Check sheet for the modelled part. Datum: model origin and axes. Units: mm. A direction names the side the tool comes from. Give positions to 0.01 mm unless a question says otherwise; leave off trailing zeros. Order: outer loops, then holes, each group sorted by start corner. A loop starts at its lowest first (then second) coordinate and runs counter-clockwise, first axis right, second up.
```python
from build123d import *

# Parameters (mm, degrees)
BOSS_EXTRUDE1_DEPTH = 3
CUT_EXTRUDE1_REACH  = 77.661
SKETCH1_3_R         = 1.25
BOSS_EXTRUDE2_START = 8.86
BOSS_EXTRUDE2_DEPTH = 8.86
BOSS_EXTRUDE3_START = 1.5
SKETCH1_5_R         = 3.21
SKETCH1_5_R_2       = 1.25
BOSS_EXTRUDE3_DEPTH = 1.5
SKETCH2_W           = 12.28
SKETCH2_H           = 8.73
CUT_EXTRUDE2_DEPTH  = 3
SKETCH3_R           = 1.6
BOSS_EXTRUDE4_DEPTH = 3
FILLET1_R           = 1
FILLET2_R           = 1


with BuildPart() as part:
    # Sketch1 → Boss-Extrude1 (new body)
    with BuildSketch(Plane(origin=(0, 0, 0), x_dir=(1, 0, 0), z_dir=(0, 1, 0))):
        with BuildLine():
            Line((3.81, 3), (49.09, 3))
            ThreePointArc((49.09, 3), (53.90539718, 1.00539718), (55.9, -3.81))
            Line((55.9, -3.81), (55.9, -44.09))
            ThreePointArc((55.9, -44.09), (53.90539718, -48.90539718), (49.09, -50.9))
            Line((49.09, -50.9), (3.81, -50.9))
            ThreePointArc((3.81, -50.9), (-1.00539718, -48.90539718), (-3, -44.09))
            Line((-3, -44.09), (-3, -3.81))
            ThreePointArc((-3, -3.81), (-1.00539718, 1.00539718), (3.81, 3))
        make_face()
    extrude(amount=-BOSS_EXTRUDE1_DEPTH)

    # Sketch1_3 → Cut-Extrude1 (cut, up to next)
    with BuildSketch(Plane(origin=(0, 0, 0), x_dir=(1, 0, 0), z_dir=(0, 1, 0)), mode=Mode.PRIVATE) as cut_extrude1_sk1:
        with Locations(Location((3.81, -3.81, 0), (0, 0, 270))):
            Circle(SKETCH1_3_R)
    cut_extrude1_tool1 = extrude(cut_extrude1_sk1.sketch, amount=-CUT_EXTRUDE1_REACH, mode=Mode.PRIVATE) & part.part
    # Sketch1_3 → Cut-Extrude1 (cut, up to next)
    with BuildSketch(Plane(origin=(0, 0, 0), x_dir=(1, 0, 0), z_dir=(0, 1, 0)), mode=Mode.PRIVATE) as cut_extrude1_sk2:
        with Locations(Location((3.81, -44.09, 0), (0, 0, 270))):
            Circle(SKETCH1_3_R)
    cut_extrude1_tool2 = extrude(cut_extrude1_sk2.sketch, amount=-CUT_EXTRUDE1_REACH, mode=Mode.PRIVATE) & part.part
    # Sketch1_3 → Cut-Extrude1 (cut, up to next)
    with BuildSketch(Plane(origin=(0, 0, 0), x_dir=(1, 0, 0), z_dir=(0, 1, 0)), mode=Mode.PRIVATE) as cut_extrude1_sk3:
        with Locations(Location((49.09, -44.09, 0), (0, 0, 270))):
            Circle(SKETCH1_3_R)
    cut_extrude1_tool3 = extrude(cut_extrude1_sk3.sketch, amount=-CUT_EXTRUDE1_REACH, mode=Mode.PRIVATE) & part.part
    # Sketch1_3 → Cut-Extrude1 (cut, up to next)
    with BuildSketch(Plane(origin=(0, 0, 0), x_dir=(1, 0, 0), z_dir=(0, 1, 0)), mode=Mode.PRIVATE) as cut_extrude1_sk4:
        with Locations(Location((49.09, -3.81, 0), (0, 0, 270))):
            Circle(SKETCH1_3_R)
    cut_extrude1_tool4 = extrude(cut_extrude1_sk4.sketch, amount=-CUT_EXTRUDE1_REACH, mode=Mode.PRIVATE) & part.part
    add(cut_extrude1_tool1.solids().sort_by_distance((3.81, 0, 3.81))[0], mode=Mode.SUBTRACT)
    add(cut_extrude1_tool2.solids().sort_by_distance((3.81, 0, 44.09))[0], mode=Mode.SUBTRACT)
    add(cut_extrude1_tool3.solids().sort_by_distance((49.09, 0, 44.09))[0], mode=Mode.SUBTRACT)
    add(cut_extrude1_tool4.solids().sort_by_distance((49.09, 0, 3.81))[0], mode=Mode.SUBTRACT)

    # Sketch1_4 → Boss-Extrude2 (add)
    with BuildSketch(Plane(origin=(0, 0, 0), x_dir=(1, 0, 0), z_dir=(0, 1, 0)).offset(BOSS_EXTRUDE2_START)):
        with BuildLine():
            ThreePointArc((-3, -3.81), (-1.00539718, 1.00539718), (3.81, 3))
            Line((3.81, 3), (49.09, 3))
            ThreePointArc((49.09, 3), (53.90539718, 1.00539718), (55.9, -3.81))
            Line((55.9, -3.81), (55.9, -44.09))
            ThreePointArc((55.9, -44.09), (53.90539718, -48.90539718), (49.09, -50.9))
            Line((49.09, -50.9), (3.81, -50.9))
            ThreePointArc((3.81, -50.9), (-1.00539718, -48.90539718), (-3, -44.09))
            Line((-3, -44.09), (-3, -3.81))
        make_face()
        with BuildLine():
            Line((52.9, -3.81), (52.9, -44.09))
            ThreePointArc((52.9, -44.09), (51.784076836, -46.784076836), (49.09, -47.9))
            Line((49.09, -47.9), (3.81, -47.9))
            ThreePointArc((3.81, -47.9), (1.115923164, -46.784076836), (0, -44.09))
            Line((0, -44.09), (0, -3.81))
            ThreePointArc((0, -3.81), (1.115923164, -1.115923164), (3.81, 0))
            Line((3.81, 0), (49.09, 0))
            ThreePointArc((49.09, 0), (51.784076836, -1.115923164), (52.9, -3.81))
        make_face(mode=Mode.SUBTRACT)
    extrude(amount=-BOSS_EXTRUDE2_DEPTH)

    # Sketch1_5 → Boss-Extrude3 (add)
    # profile 1 of 4: a face of its own
    with BuildSketch(Plane(origin=(0, 0, 0), x_dir=(1, 0, 0), z_dir=(0, 1, 0)).offset(BOSS_EXTRUDE3_START)):
        with Locations(Location((49.09, -3.81, 0), (0, 0, 90))):
            Circle(SKETCH1_5_R)
        with Locations(Location((49.09, -3.81, 0), (0, 0, 270))):
            Circle(SKETCH1_5_R_2, mode=Mode.SUBTRACT)
    # profile 2 of 4: a face of its own
    with BuildSketch(Plane(origin=(0, 0, 0), x_dir=(1, 0, 0), z_dir=(0, 1, 0)).offset(BOSS_EXTRUDE3_START)):
        with Locations(Location((49.09, -44.09, 0), (0, 0, 90))):
            Circle(SKETCH1_5_R)
        with Locations(Location((49.09, -44.09, 0), (0, 0, 270))):
            Circle(SKETCH1_5_R_2, mode=Mode.SUBTRACT)
    # profile 3 of 4: a face of its own
    with BuildSketch(Plane(origin=(0, 0, 0), x_dir=(1, 0, 0), z_dir=(0, 1, 0)).offset(BOSS_EXTRUDE3_START)):
        with Locations(Location((3.81, -44.09, 0), (0, 0, 90))):
            Circle(SKETCH1_5_R)
        with Locations(Location((3.81, -44.09, 0), (0, 0, 270))):
            Circle(SKETCH1_5_R_2, mode=Mode.SUBTRACT)
    # profile 4 of 4: a face of its own
    with BuildSketch(Plane(origin=(0, 0, 0), x_dir=(1, 0, 0), z_dir=(0, 1, 0)).offset(BOSS_EXTRUDE3_START)):
        with Locations(Location((3.81, -3.81, 0), (0, 0, 90))):
            Circle(SKETCH1_5_R)
        with Locations(Location((3.81, -3.81, 0), (0, 0, 270))):
            Circle(SKETCH1_5_R_2, mode=Mode.SUBTRACT)
    extrude(amount=-BOSS_EXTRUDE3_DEPTH)

    # Sketch2 → Cut-Extrude2 (cut)
    with BuildSketch(Plane.XY.offset(50.9)):
        with Locations((18.5, 4.5)):
            Rectangle(SKETCH2_W, SKETCH2_H)
    extrude(amount=-CUT_EXTRUDE2_DEPTH, mode=Mode.SUBTRACT)

    # Sketch3 → Boss-Extrude4 (add)
    # profile 1 of 2: a face of its own
    with BuildSketch(Plane.XZ.offset(3)):
        with BuildLine():
            Line((55.9, 18.95), (62, 18.95))
            ThreePointArc((62, 18.95), (64.757716447, 20.092283553), (65.9, 22.85))
            Line((65.9, 22.85), (65.9, 25.05))
            ThreePointArc((65.9, 25.05), (64.757716447, 27.807716447), (62, 28.95))
            Line((62, 28.95), (55.9, 28.95))
            Line((55.9, 28.95), (55.9, 18.95))
        make_face()
        with Locations(Location((60.9, 23.95, 0), (0, 0, 270))):
            Circle(SKETCH3_R, mode=Mode.SUBTRACT)
    # profile 2 of 2: a face of its own
    with BuildSketch(Plane.XZ.offset(3)):
        with BuildLine():
            Line((-3, 18.95), (-9.1, 18.95))
            ThreePointArc((-9.1, 18.95), (-11.857716447, 20.092283553), (-13, 22.85))
            Line((-13, 22.85), (-13, 25.05))
            ThreePointArc((-13, 25.05), (-11.857716447, 27.807716447), (-9.1, 28.95))
            Line((-9.1, 28.95), (-3, 28.95))
            Line((-3, 28.95), (-3, 18.95))
        make_face()
        with Locations(Location((-8, 23.95, 0), (0, 0, 270))):
            Circle(SKETCH3_R, mode=Mode.SUBTRACT)
    extrude(amount=-BOSS_EXTRUDE4_DEPTH)

    # Fillet1
    fillet1_edges = [part.edges().sort_by_distance(p)[0] for p in [
        (58.95, 0, 28.95),
        (64.757716447, 0, 27.807716447),
        (65.9, 0, 23.95),
        (64.757716447, 0, 20.092283553),
        (58.95, 0, 18.95),
    ]]
    fillet(fillet1_edges, radius=FILLET1_R)

    # Fillet2
    fillet2_edges = [part.edges().sort_by_distance(p)[0] for p in [
        (-6.05, 0, 18.95),
        (-11.857716447, 0, 20.092283553),
        (-13, 0, 23.95),
        (-11.857716447, 0, 27.807716447),
        (-6.05, 0, 28.95),
    ]]
    fillet(fillet2_edges, radius=FILLET2_R)


solid = part.part
```
(1) Release check for a two-part mould opening along X. For faces 1 (the face through (64.727, -2.014, 20.062)), 2 (the face through (-9, -1.5, 25.2)), 3 (the face through (-13, -2, 24)), 4 (the face through (59, 0, 23)) record: released by +X, released by -X, zero draft, split by the parting line, or undercut.
Response values:
face 1: released by +X
face 2: undercut
face 3: released by -X
face 4: zero draft
(2) Material ranges on L1, parallel to X at y = -0.5, z = 3.81; L2, parallel to X at y = -1.55, z = 23.95; L3, parallel to Z at x = 4, y = 0.5, recorded low to high.
Response values:
L1: x = -3 to 2.56, 5.06 to 47.84, 50.34 to 55.9
L2: x = -13 to -9.6, -6.4 to 59.3, 62.5 to 65.9
L3: z = -3 to 0, 0.61 to 2.57, 5.05 to 7.01, 40.89 to 42.85, 45.33 to 47.29, 47.9 to 50.9
(3) Cross-section at A-A on x = 60.9. Enter the section's corners in (y, z).
Response values:
outline: (-3, 18.95) - (-1, 18.95) arc R1 ccw to (0, 19.95) - (0, 22.35) - (-3, 22.35) - close; (-3, 25.55) - (0, 25.55) - (0, 27.95) arc R1 ccw to (-1, 28.95) - (-3, 28.95) - close
(4) Gauge pin test, flat ends, axial feed: pin 1 Ø1.9 at (x, z) = (3, 44) entering from +Y; pin 2 Ø1 at (y, z) = (5, 37.5) entering from +X; pin 3 Ø2 at (y, z) = (5.5, 11.5) entering from -X; pin 4 Ø1.5 at (x, z) = (49.09, 44.09) entering from -Y. Record the tip position at first contact, or that the pin passes through.
Response values:
pin 1: stops at y = 1.5
pin 2: stops at x = 55.9
pin 3: stops at x = -3
pin 4: passes through
(5) Cross-section at C-C on z = 13. Enter the section's corners in (x, y), then the cut area to 3 significant figures.
Response values:
outline: (-3, -3) - (55.9, -3) - (55.9, 8.86) - (52.9, 8.86) - (52.9, 0) - (0, 0) - (0, 8.86) - (-3, 8.86) - close
area: 230 mm2
(6) Set-up check for faces 5 (the face through (26, 4, 0)), 6 (the face through (-6, -2, 28.95)), 7 (the face through (18, 0.135, 49)), 8 (the face through (59, -2, 28.95)): record each of +Z, -Z, +X, -X, +Y, -Y from which the full face is reachable in a straight line by a thin tool's end or side.
Response values:
face 5: +Y
face 6: +Z, -X, +Y, -Y
face 7: +Z, +Y
face 8: +Z, +X, +Y, -Y
(7) Cross-section at D-D on y = 5.5. Enter the section's corners in (x, z), then the cut area to 3 significant figures.
Response values:
outline: (-3, 3.81) arc R6.81 ccw to (3.81, -3) - (49.09, -3) arc R6.81 ccw to (55.9, 3.81) - (55.9, 44.09) arc R6.81 ccw to (49.09, 50.9) - (24.64, 50.9) - (24.64, 47.9) - (49.09, 47.9) arc R3.81 cw to (52.9, 44.09) - (52.9, 3.81) arc R3.81 cw to (49.09, 0) - (3.81, 0) arc R3.81 cw to (0, 3.81) - (0, 44.09) arc R3.81 cw to (3.81, 47.9) - (12.36, 47.9) - (12.36, 50.9) - (3.81, 50.9) arc R6.81 ccw to (-3, 44.09) - close
area: 577 mm2
(8) Cross-section at B-B on x = 17. Enter the section's corners in (y, z) (3 decimals).
Response values:
outline: (-3, -3) - (8.86, -3) - (8.86, 0) - (0, 0) - (0, 47.9) - (0.135, 47.9) - (0.135, 50.9) - (-3, 50.9) - close
